Autodesk Inventor part; units mm, degrees
ref_plane "YZ Plane" through (0, 0, 0) normal (1, 0, 0) x (0, 1, 0)
ref_plane "XZ Plane" through (0, 0, 0) normal (0, 1, 0) x (-1, 0, 0)
ref_plane "XY Plane" through (0, 0, 0) normal (0, 0, 1) x (1, 0, 0)
sketch "Sketch2" plane through (0, 0, 0) normal (0, 1, 0) x (-1, 0, 0)
  circle A0 centre (0, 0) radius 80 construction
  line L0 (77.2741, 20.7055) -> (103.156, -75.8871)
  line L1 (-77.2741, -20.7055) -> (-51.3922, -117.2981)
  line L2 (103.156, -75.8871) -> (-51.3922, -117.2981) construction
  line L3 (103.156, -75.8871) -> (103.156, -235.8871) construction
  line L4 (103.156, -235.8871) -> (-51.3922, -194.476) construction
  line L5 (-51.3922, -117.2981) -> (-51.3922, -194.476)
  circle A1 centre (0, -311.7741) radius 80 construction
  line L6 (-51.3922, -194.476) -> (-77.2741, -291.0686)
  line L7 (103.156, -235.8871) -> (77.2741, -332.4796)
  arc A2 (77.2741, 20.7055) -> (-77.2741, -20.7055) centre (0, 0) ccw
  arc A3 (-77.2741, -291.0686) -> (77.2741, -332.4796) centre (0, -311.7741) ccw
  circle A4 centre (0, 0) radius 7.5
  circle A5 centre (0, -311.7741) radius 7.5
  line L8 (83.156, -48.3871) -> (-31.844, -48.3871)
  line L9 (-31.844, -48.3871) -> (-31.844, -263.3871)
  line L10 (-31.844, -263.3871) -> (83.156, -263.3871)
  line L11 (83.156, -263.3871) -> (83.156, -48.3871)
  arc A6 (103.156, -235.8871) -> (103.156, -75.8871) centre (-201.516, -155.8871) ccw
  circle A7 centre (98.32, -155.8871) radius 7.5
  point P0 (103.156, -155.8871)
  point P1 (83.156, -155.8871)
  dimension "d0" = 160
  dimension "d1" = 100
  dimension "d2" = 100
  dimension "d3" = 160
  dimension "d4" = 160
  dimension "d5" = 160
  dimension "d6" = 75
  dimension "d7" = 75
  dimension "d8" = 160
  dimension "d9" = 100
  dimension "d10" = 100
  dimension "d11" = 15
  dimension "d12" = 15
  dimension "d13" = 115
  dimension "d14" = 215
  dimension "d15" = 20
  dimension "d39" = 315
  dimension "d40" = 15
  dimension "d41" = 15.164
extrude "Extrusion1" add sketch "Sketch2" along normal blind 339
sketch "Sketch5" plane through (31.844, 0, -48.3871) normal (-1, 0, 0) x (0, 0, 1)
  line L0 (0, 0) -> (-215, 0) construction
  line L1 (0, 0) -> (0, 339) construction
  line L2 (-215, 339) -> (0, 339) construction
  line L3 (-215, 0) -> (-215, 339) construction
  line L4 (-68.911, 0) -> (27.6815, 0) construction
  line L5 (0, 339) -> (-19, 339) construction
  line L6 (-19, 339) -> (-19, 0) construction
  line L7 (-19, 0) -> (0, 0) construction
  line L8 (0, 0) -> (0, 339) construction
  line L9 (-146.089, 339) -> (-242.6815, 339) construction
  line L10 (-215, 0) -> (-196, 0) construction
  line L11 (-196, 0) -> (-196, 339) construction
  line L12 (-196, 339) -> (-215, 339) construction
  line L13 (-215, 339) -> (-215, 0) construction
  circle A0 centre (-205.5, 329) radius 2.5
  circle A1 centre (-205.5, 10) radius 2.5
  circle A2 centre (-9.5, 329) radius 2.5
  circle A3 centre (-9.5, 10) radius 2.5
  point P0 (-205.5, 0)
  point P1 (-205.5, 339)
  point P2 (-9.5, 0)
  point P3 (-9.5, 339)
  dimension "d52" = 19
  dimension "d53" = 19
  dimension "d54" = 5
  dimension "d55" = 10
  dimension "d56" = 5
  dimension "d57" = 10
  dimension "d58" = 5
  dimension "d59" = 5
  dimension "d60" = 10
  dimension "d61" = 10
extrude "Extrusion4" cut sketch "Sketch5" along normal through all both and the other way through all
sketch "Sketch6" plane through (0, 339, 0) normal (0, 1, 0) x (1, 0, 0)
  line L0 (-28.5041, 0.1269) -> (24.6218, 14.362) construction
  line L1 (-103.156, 75.8871) -> (-77.2741, -20.7055) construction
  line L2 (-77.2741, -20.7055) -> (-103.156, 75.8871) construction
  line L3 (-103.156, 75.8871) -> (51.3922, 117.2981) construction
  line L4 (-25.8819, 96.5926) -> (-1.9411, 7.2444) construction
  circle A0 centre (-28.5041, 0.1269) radius 2.5
  circle A1 centre (24.6218, 14.362) radius 2.5
  line L5 (-103.156, 235.8871) -> (-77.2741, 332.4796) construction
  line L6 (51.3922, 194.476) -> (77.2741, 291.0686) construction
  line L7 (-103.156, 235.8871) -> (51.3922, 194.476) construction
  line L8 (-25.8819, 215.1815) -> (-1.9411, 304.5297) construction
  line L9 (24.6218, 297.4122) -> (-28.5041, 311.6472) construction
  circle A2 centre (-28.5041, 311.6472) radius 2.5
  circle A3 centre (24.6218, 297.4122) radius 2.5
  point P0 (0, 0)
  dimension "d64" = 55
  dimension "d65" = 92.5
  dimension "d66" = 5
  dimension "d67" = 5
  dimension "d68" = 92.5
  dimension "d69" = 5
  dimension "d70" = 5
  dimension "d71" = 55
extrude "Extrusion5" cut sketch "Sketch6" against normal blind 25
sketch "Sketch9" plane through (-77.2741, 0, 20.7055) normal (-0.9659258, 0, 0.258819) x (0.258819, 0, 0.9659258)
  line L0 (-10, 314) -> (-5, 314)
  line L1 (-10, 339) -> (-5, 339)
  line L2 (-10, 314) -> (-5, 314)
  line L3 (-10, 339) -> (-5, 339)
  line L4 (-12.5, 334) -> (-2.5, 334)
  line L5 (-2.5, 334) -> (-2.5, 329)
  line L6 (-2.5, 329) -> (-12.5, 329)
  line L7 (-12.5, 329) -> (-12.5, 334)
  point P0 (0, 0)
  point P1 (-7.5, 334)
  point P2 (-7.5, 339)
  dimension "d80" = 10
  dimension "d81" = 5
  dimension "d82" = 5
extrude "Extrusion7" cut sketch "Sketch9" against normal through all
sketch "Sketch10" plane through (-103.156, 0, -235.8871) normal (-0.9659258, 0, -0.258819) x (-0.258819, 0, 0.9659258)
  line L0 (-95, 314) -> (-90, 314)
  line L1 (-95, 339) -> (-90, 339)
  line L2 (-97.5, 334) -> (-87.5, 334)
  line L3 (-87.5, 334) -> (-87.5, 329)
  line L4 (-87.5, 329) -> (-97.5, 329)
  line L5 (-97.5, 329) -> (-97.5, 334)
  point P0 (201.1507, 0)
  point P1 (-92.5, 334)
  point P2 (-92.5, 339)
  dimension "d85" = 10
  dimension "d86" = 5
  dimension "d87" = 5
extrude "Extrusion8" cut sketch "Sketch10" against normal through all
properties part number "TA001" material "ABS Plastic"
Model file for the job. Use its own axes, mm. A direction names the side the tool comes from. Give positions to 0.01 mm unless a question says otherwise; leave off trailing zeros. Order: outer loops, then holes, each group sorted by start corner. A loop starts at its lowest first (then second) coordinate and runs counter-clockwise, first axis right, second up. Notation, with made-up numbers: M 26.25,46 L 73.25,46 A24 ccw 73.25,64 Z; hole C -29.75,53 d4. An arc over 180 degrees is marked long. Write item = value, one per line.
Q1. Cut at A-A, the plane x = -20.5. List the corners of the cut face in (y, z), then the cut area to 3 significant figures.
Derived:
outline = M 0,-389.1 L 339,-389.1 L 339,-263.39 L 0,-263.39 Z; M 0,-48.39 L 339,-48.39 L 339,77.33 L 0,77.33 Z; hole M 329,-314.68 L 334,-314.68 L 334,-304.33 L 329,-304.33 Z; hole M 329,-7.45 L 334,-7.45 L 334,2.9 L 329,2.9 Z
area = 85,100 mm2
Q2. Cut at B-B, the plane z = -83. List the corners of the cut face in (x, y).
Derived:
outline = M -104.94,0 L -83.16,0 L -83.16,339 L -104.94,339 Z; M 31.84,0 L 60.58,0 L 60.58,339 L 31.84,339 Z
Q3. Flat gauge pins, fed straight in: pin 1 (6 mm diameter, centred on y = 10, z = -57.89, fed in from -X); pin 2 (10 mm diameter, centred on x = 49.5, y = 205, fed in from +Z); pin 3 (4 mm diameter, centred on y = 127.5, z = -77, fed in from -X); pin 4 (13.5 mm diameter, centred on x = 0, z = 0, fed in from +Y). Where does each tip first touch, or does it go through?
Derived:
pin_1 = -99.14
pin_2 = 66.48
pin_3 = -103.96
pin_4 = through
Q4. Drill centre lines: line 1 (Z direction, x = 44.5, y = 10); line 2 (X direction, y = 60.5, z = -69.5); line 3 (Y direction, x = -55.5, z = -320). Where is each one in solid material? Low to high. Write a range as [from, to].
Derived:
line_1 = [-378.26, -256.39], [-251.39, -60.39], [-55.39, 66.48]
line_2 = [-101.44, -83.16], [31.84, 64.2]
line_3 = [0, 329], [334, 339]
Q5. Two-plate mould, pull along X, no slides. Class faces 4 (the flat face through (-90.4, 167.1, -283.5)), 5 (the flat face through (40.912, 331.465, -298.224)), 6 (the flat face through (49, 0, -153)), 7 (the flat face through (51.392, 167, -155)): pulls with the +X half, pulls with the -X half, needs draft (parallel to the pull), parting line crosses it, or undercut.
Derived:
face_4 = pulls with the -X half
face_5 = undercut
face_6 = needs draft
face_7 = pulls with the +X half
Q6. Cut at C-C, the plane x = -65. List the corners of the cut face in (y, z).
Derived:
outline = M 0,-358.41 L 339,-358.41 L 339,-263.39 L 0,-263.39 Z; M 0,-48.39 L 339,-48.39 L 339,46.64 L 0,46.64 Z; hole M 329,-326.6 L 334,-326.6 L 334,-316.25 L 329,-316.25 Z; hole M 329,4.48 L 334,4.48 L 334,14.83 L 329,14.83 Z
Q7. Tool access for faces 1 (the flat face through (64.514, 167.127, -68.326)), 2 (the flat face through (31.844, 167, -154)), 3 (the flat face through (-3.04, 329, -304.75)): list every direction of +Z, -Z, +X, -X, +Y, -Y with a clear straight run to the whole face (end or side of a thin tool).
Derived:
face_1 = +X, +Y, -Y
face_2 = +Y, -Y
face_3 = none
